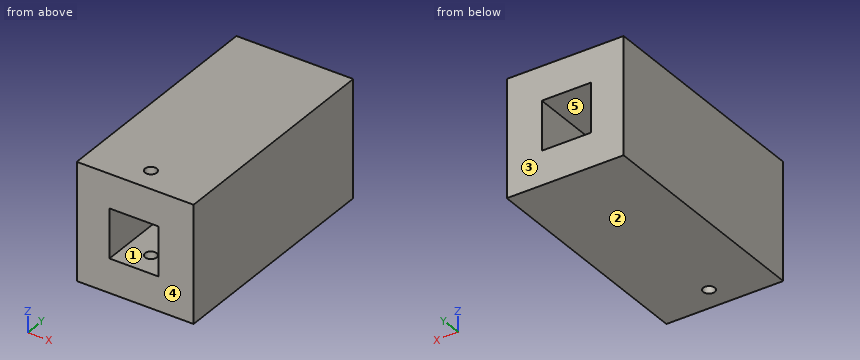
from build123d import *

# Parameters (mm, degrees)
F0_W          = 63.5
F0_H          = 127
F1_DEPTH      = 63.5
F2_W          = 26.67
F2_H          = 26.67
F3_DEPTH      = 127.001
F4_R          = 3.175
F5_DEPTH      = 45.086
F5_DEPTH_BACK = 25.4


with BuildPart() as f1:
    # F0 (on Top) → F1 (new body)
    with BuildSketch(Plane.XY):
        with Locations((1.295127, 30.201528)):
            Rectangle(F0_W, F0_H)
    extrude(amount=F1_DEPTH)

    # F2 (on face) → F3 (cut, through all)
    with BuildSketch(Plane.XZ.offset(33.298472)):
        with Locations((0.660127, 31.75)):
            Rectangle(F2_W, F2_H)
    extrude(amount=-F3_DEPTH, mode=Mode.SUBTRACT)

    # F4 (on face) → F5 (cut, two sides)
    with BuildSketch(Plane(origin=(0, 0, 45.085), x_dir=(1, 0, 0), z_dir=(0, 0, -1))) as f5_sk:
        with Locations((1.168133, 20.599107)):
            Circle(F4_R)
    extrude(amount=F5_DEPTH, mode=Mode.SUBTRACT)
    extrude(f5_sk.sketch, amount=-F5_DEPTH_BACK, mode=Mode.SUBTRACT)


solid = f1.part
Here's how the part is built. I have some questions about the finished solid (model axes, mm). Face numbers are marked on the shaded views. A direction names the side the tool comes from. Coordinates: 2 decimals unless noted, no trailing zeros. Loops run counter-clockwise (first coordinate to the right, second up) from the corner with the lowest first, then second, coordinate; pieces in that order, holes last.
1. Imagine slicing it at C-C, the plane y = 21. Please give me the cut outline in (x, z) (3 decimals).
2. Imagine slicing it at B-B, the plane z = 39. Please give me the cut outline in (x, y), and give its area (3 significant figures).
3. For P1, Ø10, axis at x = 1.17, y = -20.6, coming from the +Z side; P2, Ø4, axis at x = 1.17, y = -20.6, coming from the -Z side, each with a flat end and sliding along its axis, tell me the tip position at first contact or that it passes through.
4. For the marked faces 4 and 5, which set-ups out of +Z, -Z, +X, -X, +Y, -Y let a thin tool reach every point of the face, with its end or its side?
5. I need wall thicknesses on L1, parallel to X at y = 2, z = 29; L2, parallel to Z at x = 7, y = 38.5 (3 decimals). Which ranges of each line are inside material? Lowest first, please.
6. Imagine slicing it at A-A, the plane x = -7. Please give me the cut outline in (y, z) (3 decimals), and give its area (3 significant figures).
7. If we mould it in two halves opening along Z, with no side actions, what happens to the marked faces 1, 2 and 3? For each: pulls with the +Z half, pulls with the -Z half, needs draft (parallel to the pull), parting line crosses it, or undercut.
Taken from the geometry:
1. outline: (-30.455, 0) - (33.045, 0) - (33.045, 63.5) - (-30.455, 63.5) - close; hole (-12.675, 18.415) - (13.995, 18.415) - (13.995, 45.085) - (-12.675, 45.085) - close
2. outline: (-30.45, -33.3) - (-12.67, -33.3) - (-12.67, 93.7) - (-30.45, 93.7) - close; (14, -33.3) - (33.05, -33.3) - (33.05, 93.7) - (14, 93.7) - close
2. area: 4,680 mm2
3. P1: stops at z = 63.5
3. P2: passes through
4. face 4: +Z, -Z, +X, -X, -Y
4. face 5: +Y, -Y
5. L1: x = -30.45 to -12.67, 14 to 33.05
5. L2: z = 0 to 18.415, 45.085 to 63.5
6. outline: (-33.298, 0) - (93.702, 0) - (93.702, 18.415) - (-33.298, 18.415) - close; (-33.298, 45.085) - (93.702, 45.085) - (93.702, 63.5) - (-33.298, 63.5) - close
6. area: 4,680 mm2
7. face 1: undercut
7. face 2: pulls with the -Z half
7. face 3: needs draft
